from build123d import *

# Parameters (mm, degrees)
SKIZZE1_W                       = 20
SKIZZE1_H                       = 20
SKIZZE1_W_2                     = 17
SKIZZE1_H_2                     = 17
AUFSATZ_LINEAR_AUSTRAGEN1_DEPTH = 250
SKIZZE2_R                       = 3.25
SCHNITT_LINEAR_AUSTRAGEN1_DEPTH = 15
SKIZZE3_R                       = 3.25
SCHNITT_LINEAR_AUSTRAGEN2_DEPTH = 15


with BuildPart() as part:
    # Skizze1 → Aufsatz-Linear austragen1 (new, symmetric)
    with BuildSketch(Plane.XY):
        Rectangle(SKIZZE1_W, SKIZZE1_H)
        Rectangle(SKIZZE1_W_2, SKIZZE1_H_2, mode=Mode.SUBTRACT)
    extrude(amount=AUFSATZ_LINEAR_AUSTRAGEN1_DEPTH, both=True)

    # Skizze2 → Schnitt-Linear austragen1 (cut, symmetric)
    with BuildSketch(Plane(origin=(0, 0, 0), x_dir=(1, 0, 0), z_dir=(0, 1, 0))):
        with Locations((0, -220)):
            Circle(SKIZZE2_R)
        with Locations((0, 220)):
            Circle(SKIZZE2_R)
    extrude(amount=SCHNITT_LINEAR_AUSTRAGEN1_DEPTH, both=True, mode=Mode.SUBTRACT)

    # Skizze3 → Schnitt-Linear austragen2 (cut, symmetric)
    with BuildSketch(Plane(origin=(0, 0, 0), x_dir=(0, 0, -1), z_dir=(1, 0, 0))):
        with Locations((-240, 0)):
            Circle(SKIZZE3_R)
        with Locations((240, 0)):
            Circle(SKIZZE3_R)
    extrude(amount=SCHNITT_LINEAR_AUSTRAGEN2_DEPTH, both=True, mode=Mode.SUBTRACT)


solid = part.part
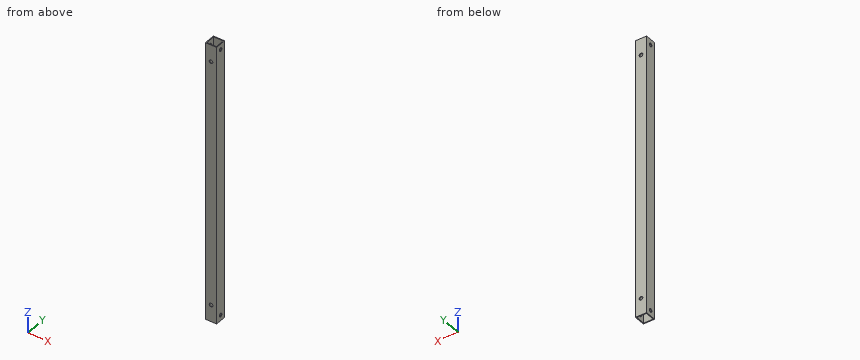
CAD build for the part. Positions are in the model's coordinates, mm. Give positions to 0.01 mm unless a question says otherwise; leave off trailing zeros. Write each loop counter-clockwise with the first axis right and the second up, starting at its lowest first coordinate (ties: lowest second). Pieces come first, ordered by that corner, then holes. Notation, with made-up numbers: (53.5, 28.5) - (58.5, 28.5) arc R30 ccw to (58.5, 51.5) - close; hole circle Ø10 at (10.25, 43.25). An arc over 180 degrees is marked (long way). Answer as CSV lines item,"result".
Q1. Band-saw the part on B-B (y = 0). Give the cut face in (x, z), and give its area (3 significant figures).
Result set:
outline,"(-10, -250) - (-8.5, -250) - (-8.5, -243.25) - (-10, -243.25) - close; (-10, -236.75) - (-8.5, -236.75) - (-8.5, 236.75) - (-10, 236.75) - close; (-10, 243.25) - (-8.5, 243.25) - (-8.5, 250) - (-10, 250) - close; (8.5, -250) - (10, -250) - (10, -243.25) - (8.5, -243.25) - close; (8.5, -236.75) - (10, -236.75) - (10, 236.75) - (8.5, 236.75) - close; (8.5, 243.25) - (10, 243.25) - (10, 250) - (8.5, 250) - close"
area,"1,460 mm²"
Q2. Band-saw the part on A-A (x = 0). Give the cut face in (y, z), and give its area (3 significant figures).
Result set:
outline,"(-10, -250) - (-8.5, -250) - (-8.5, -223.25) - (-10, -223.25) - close; (-10, -216.75) - (-8.5, -216.75) - (-8.5, 216.75) - (-10, 216.75) - close; (-10, 223.25) - (-8.5, 223.25) - (-8.5, 250) - (-10, 250) - close; (8.5, -250) - (10, -250) - (10, -223.25) - (8.5, -223.25) - close; (8.5, -216.75) - (10, -216.75) - (10, 216.75) - (8.5, 216.75) - close; (8.5, 223.25) - (10, 223.25) - (10, 250) - (8.5, 250) - close"
area,"1,460 mm²"
Q3. Flat gauge pin, fed straight in: pin 1 Ø10.5 at (y, z) = (0, 240) entering from -X. Where does the tip first touch, or does it go through?
Result set:
pin 1,"x = -10"
Q4. Band-saw the part on C-C (z = -39.5). Give the cut face in (x, y).
Result set:
outline,"(-10, -10) - (10, -10) - (10, 10) - (-10, 10) - close; hole (-8.5, -8.5) - (8.5, -8.5) - (8.5, 8.5) - (-8.5, 8.5) - close"
Q5. Drill centre lines: line 1 (X direction, y = 9.25, z = 220); line 2 (Z direction, x = 0, y = 9.45); line 3 (X direction, y = 8, z = 4.5). Where is each one in solid material? Low to high. Write a range as from..to.
Result set:
line 1,"-10..-3.25, 3.25..10"
line 2,"-250..-223.25, -216.75..216.75, 223.25..250"
line 3,"-10..-8.5, 8.5..10"
